Geometry: see drawing. Coordinates: mm, zero at the bounding-box minimum. Give positions to 0.01 mm unless a question says otherwise; leave off trailing zeros. Order: outer loops, then holes, each group sorted by start corner. A loop starts at its lowest first (then second) coordinate and runs counter-clockwise, first axis right, second up. Notation, with made-up numbers: (-31, 31) - (-4, 31) arc R22 ccw to (-4, 64) - close; hole circle Ø7 at (-19.5, 41). An arc over 180 degrees is marked (long way). One line per question, with ' | ' between items. Start each with the question number.
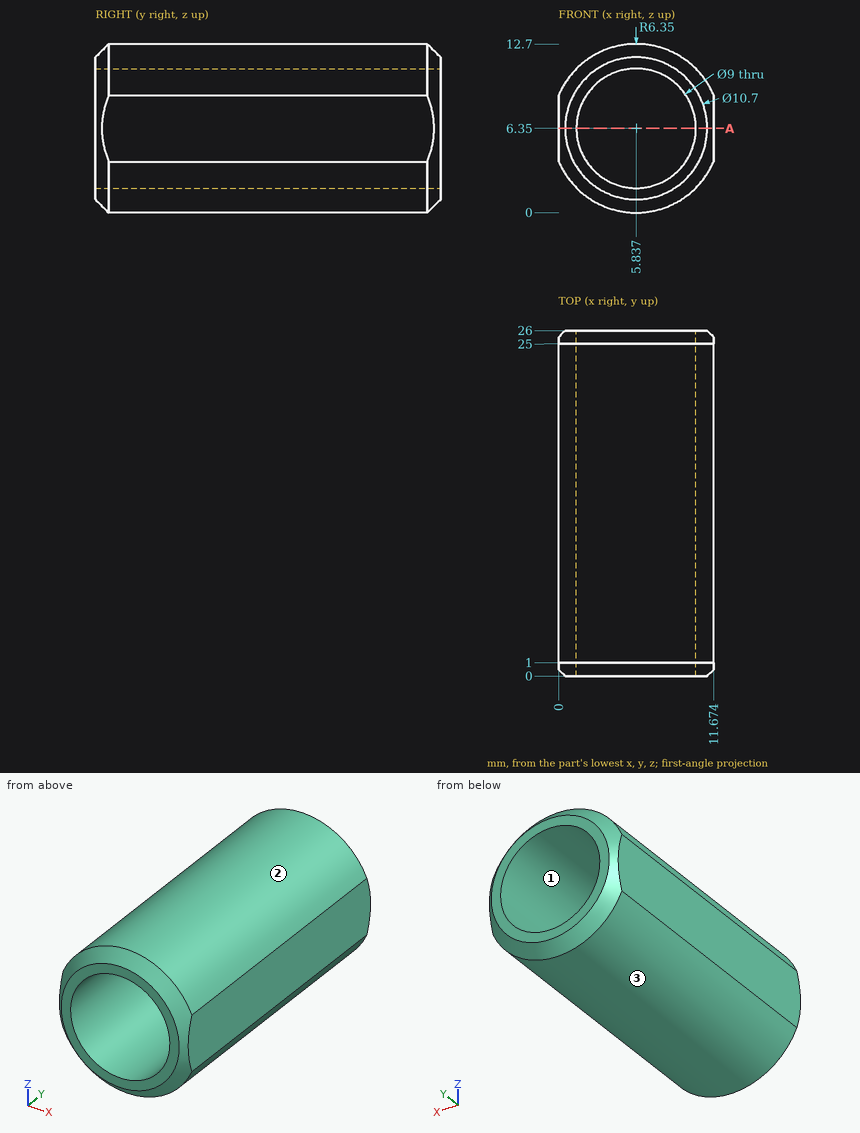
(1) Cut plane A-A, the plane z = 6.35. Return the cut outline in (x, y) (1 decimal).
(2) Contact query for flat-ended pins moving along their axis: P1, Ø3, axis at x = 1.5, y = 6.5, coming from the -Z side; P2, Ø1.5, axis at y = 22.5, z = 1.5, coming from the -X side; P3, Ø1, axis at x = 2, y = 14, coming from the -Z side. Output: stop coordinate, or through.
(3) Pull-direction query (Z, two-part tool) for the marked faces 1, 2 and 3; classes: +Z half, -Z half, draft (parallel to the pull), parting line (faces both ways), or undercut.
(4) Material intervals for line 1 along X through (y, z) = (20.5, 6.35) (1 decimal); line 2 along Z through (x, y) = (5.75, 20.75); line 3 along X through (y, z) = (23.25, 7) (1 decimal), sorted ascending. Write a range as from..to.
Results are:
1) outline: (0, 0.5) - (0.5, 0) - (1.3, 0) - (1.3, 26) - (0.5, 26) - (0, 25.5) - close; (10.3, 0) - (11.2, 0) - (11.7, 0.5) - (11.7, 25.5) - (11.2, 26) - (10.3, 26) - close
2) P1: z = 0.67 | P2: x = 0.99 | P3: z = 0.95
3) face 1: undercut | face 2: +Z half | face 3: -Z half
4) line 1: 0..1.3, 10.3..11.7 | line 2: 0..1.85, 10.85..12.7 | line 3: 0..1.4, 10.3..11.7
